Input: part model. Units: mm. Frame: model coordinates. A direction names the side the tool comes from. Give positions to 0.01 mm unless a question says otherwise; leave off trailing zeros. Write each loop counter-clockwise with the first axis right and the second up, starting at its lowest first coordinate (ties: lowest second). Pieces come first, ordered by that corner, then holes.
Autodesk Inventor part; units mm, degrees
ref_plane "YZ Plane" through (0, 0, 0) normal (1, 0, 0) x (0, 1, 0)
ref_plane "XZ Plane" through (0, 0, 0) normal (0, 1, 0) x (-1, 0, 0)
ref_plane "XY Plane" through (0, 0, 0) normal (0, 0, 1) x (1, 0, 0)
sketch "Sketch1" plane through (0, 0, 0) normal (0, 1, 0) x (-1, 0, 0)
  line L0 (0, 0) -> (8, 0)
  line L1 (8, 0) -> (8, 85)
  line L2 (8, 85) -> (0, 85)
  line L3 (0, 85) -> (0, 0)
  dimension "d0" = 8
  dimension "d1" = 85
extrude "Extrusion1" add sketch "Sketch1" along normal blind 4
sketch "Sketch2" plane through (0, 4, 0) normal (0, 1, 0) x (1, 0, 0)
  line L0 (-8, -85) -> (0, -85)
  line L1 (-4, -85) -> (-11, -85)
  line L2 (-11, -85) -> (-11, -95)
  line L3 (-11, -95) -> (-4, -95)
  line L4 (-4, -95) -> (-4, -85)
  point P0 (0, 0)
  dimension "d4" = 7
  dimension "d5" = 10
extrude "Extrusion2" add sketch "Sketch2" against normal blind 4
sketch "Sketch3" plane through (0, 4, 0) normal (0, 1, 0) x (1, 0, 0)
  line L0 (-4, -85) -> (-4, -95)
  line L1 (-4, -85) -> (3, -85)
  line L2 (3, -85) -> (3, -95)
  line L3 (3, -95) -> (-4, -95)
  line L4 (-4, -95) -> (-4, -85)
  point P0 (0, 0)
  dimension "d8" = 7
  dimension "d9" = 10
extrude "Extrusion3" add sketch "Sketch3" against normal blind 4
sketch "Sketch5" plane through (0, 4, 0) normal (0, 1, 0) x (1, 0, 0)
  line L0 (-11, -95) -> (-11, -85)
  line L1 (-11, -95) -> (-4, -95)
  line L2 (-4, -95) -> (-4, -90)
  line L3 (-4, -90) -> (-11, -90)
  line L4 (-11, -90) -> (-11, -95)
  circle A0 centre (-4, -90) radius 2
  point P0 (0, 0)
  dimension "d14" = 7
  dimension "d15" = 5
  dimension "d16" = 4
extrude "Extrusion4" cut sketch "Sketch5" against normal blind 4 contours A0 L2 L3 | L3 L2 A0
properties part number "seddd"
Q1. Access query for faces 1 (the flat face through (0, 2, 43)), 2 (the flat face through (-4, 2, 0)), 3 (the flat face through (-9, 2, 85)). Directions: +Z, -Z, +X, -X, +Y, -Y. A direction counts if a zero-diameter tool reaches every point of the face in a straight line with its end or side. Return the directions, or none.
Q2. Section A-A, the plane z = 90. Return the cut outline in (x, y).
Q3. Material intervals for line 1 along Z through (x, y) = (-4, 2.15); line 2 along X through (y, z) = (1.75, 90); line 3 along Z through (x, y) = (-8.25, 2.35), sorted ascending.
Q4. Section B-B, the plane x = -4. Return the cut outline in (y, z).
Q5. Pin query (flat end, axial travel): pin 1 (1.5 mm diameter, centred on x = -9, y = 2, fed in from -Z); pin 2 (1.2 mm diameter, centred on y = 2, z = 48, fed in from +X). Return the tip coordinate at first contact, or that it passes through.
Q6. Mould query, pull axis Z, two halves, no side actions, for faces 4 (the flat face through (-4, 4, 47)), 5 (the cylindrical face through (-4, 2, 88)), 6 (the flat face through (-4, 2, 95)). Classes: +Z half, -Z half, draft (parallel to the pull), parting line (faces both ways), or undercut.
Q7. Section C-C, the plane y = 3.1. Return the cut outline in (x, z), then the cut area to 3 significant figures.
Solutions:
1. face 1: -Z, +X, +Y, -Y
1. face 2: -Z, +X, -X, +Y, -Y
1. face 3: -Z, -X, +Y, -Y
2. outline: (-11, 0) - (-6, 0) - (-6, 4) - (-11, 4) - close; (-2, 0) - (3, 0) - (3, 4) - (-2, 4) - close
3. line 1: z = 0 to 88, 92 to 95
3. line 2: x = -11 to -6, -2 to 3
3. line 3: z = 85 to 95
4. outline: (0, 0) - (4, 0) - (4, 88) - (0, 88) - close; (0, 92) - (4, 92) - (4, 95) - (0, 95) - close
5. pin 1: stops at z = 85
5. pin 2: stops at x = 0
6. face 4: draft
6. face 5: undercut
6. face 6: +Z half
7. outline: (-11, 85) - (-8, 85) - (-8, 0) - (0, 0) - (0, 85) - (3, 85) - (3, 95) - (-11, 95) - close; hole circle Ø4 at (-4, 90)
7. area: 807 mm2
